For this review, take the finished solid that the model builds, in its own axes (mm). Face numbers are marked on the shaded views. A direction names the side the tool comes from. Give positions to 0.01 mm unless a question says otherwise; leave off trailing zeros. Loops run counter-clockwise (first coordinate to the right, second up) from the corner with the lowest first, then second, coordinate; pieces in that order, holes last.
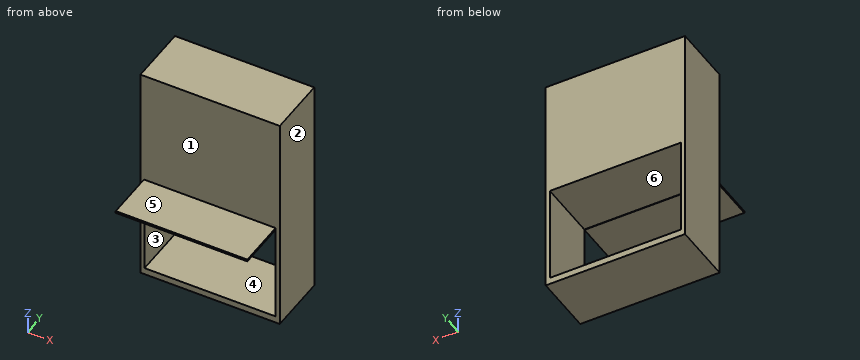
```python
from build123d import *

# Parameters (mm, degrees)
F0_W      = 1295.4
F0_H      = 2082.8
F1_DEPTH  = 558.8
F3_W      = 1219.2
F3_H      = 914.4
F9_DEPTH  = 558.8
F10_W     = 1223.48994
F10_H     = 19.100845
F11_DEPTH = 457.2


with BuildPart() as f1:
    # F0 (on Front) → F1 (new body)
    with BuildSketch(Plane.XZ):
        with Locations((80.820927, 6.07419)):
            Rectangle(F0_W, F0_H)
    extrude(amount=-F1_DEPTH)

    # F3 (on face) → F9 (cut, through all)
    with BuildSketch(Plane.XZ):
        with Locations((80.820927, -514.62581)):
            Rectangle(F3_W, F3_H)
    extrude(amount=-F9_DEPTH, mode=Mode.SUBTRACT)

    # F10 (on face) → F11 (join)
    with BuildSketch(Plane.XZ):
        with Locations((77.789873, -51.771193)):
            Rectangle(F10_W, F10_H)
    extrude(amount=F11_DEPTH)


solid = f1.part
```
Item 1: Take a section at B-B on z = -599.5. Give the boundary of the cut face in (x, y), and give its area (3 significant figures).
Answer:
outline: (-566.88, 0) - (-528.78, 0) - (-528.78, 558.8) - (-566.88, 558.8) - close; (690.42, 0) - (728.52, 0) - (728.52, 558.8) - (690.42, 558.8) - close
area: 42,600 mm2
Item 2: For L1, parallel to X at y = 428, z = -648.5; L2, parallel to Z at x = 250, y = 338; L3, parallel to Y at x = 242, z = 142, list the stretches that pass through material, from the lowest coordinate up.
Answer:
L1: x = -566.88 to -528.78, 690.42 to 728.52
L2: z = -1035.33 to -971.83, -57.43 to 1047.47
L3: y = 0 to 558.8
Item 3: The part is to be moulded in two halves that separate along X. For the marked faces 1, 2 and 3, say which applies: released by +X, released by -X, zero draft, split by the parting line, or undercut.
Answer:
face 1: zero draft
face 2: released by +X
face 3: undercut
Item 4: Take a section at C-C on y = 339. Give the boundary of the cut face in (x, z), and give its area (3 significant figures).
Answer:
outline: (-566.88, -1035.33) - (728.52, -1035.33) - (728.52, 1047.47) - (-566.88, 1047.47) - close; hole (-528.78, -971.83) - (690.42, -971.83) - (690.42, -57.43) - (-528.78, -57.43) - close
area: 1,580,000 mm2
Item 5: Clearance check with flat-ended pins moving along their axes: pin 1 Ø9.5 at (y, z) = (-117.5, -48.5) entering from +X; pin 2 Ø1.9 at (x, z) = (87.5, -59.5) entering from +Y; pin 3 Ø21 at (y, z) = (-261, -49.5) entering from -X. State where each tip first meets the part, or that it passes through.
Answer:
pin 1: stops at x = 689.53
pin 2: stops at y = 0
pin 3: stops at x = -533.96
Item 6: Take a section at D-D on z = 377. Give the boundary of the cut face in (x, y).
Answer:
outline: (-566.88, 0) - (728.52, 0) - (728.52, 558.8) - (-566.88, 558.8) - close
Item 7: Tool access review of the marked faces 4, 5 and 6: name each direction out of +Z, -Z, +X, -X, +Y, -Y from which nothing blocks a thin tool from reaching the whole face with its end or side.
Answer:
face 4: +Y, -Y
face 5: +Z, +X, -X, -Y
face 6: +Y
Item 8: Take a section at A-A on x = 430. Give the boundary of the cut face in (y, z).
Answer:
outline: (-457.2, -61.32) - (0, -61.32) - (0, -57.43) - (558.8, -57.43) - (558.8, 1047.47) - (0, 1047.47) - (0, -42.22) - (-457.2, -42.22) - close; (0, -1035.33) - (558.8, -1035.33) - (558.8, -971.83) - (0, -971.83) - close
